Input: dimensioned drawing with shaded views. Units: mm. Origin: part minimum x, y, z. A direction names the side the tool comes from. Round coordinates to 2 decimals unless told otherwise and drop trailing zeros. Order: outer loops, then holes, each group sorted by start corner. A loop starts at its lowest first (then second) coordinate and runs counter-clockwise, first axis right, second up. Notation, with made-up numbers: M -31,51.25 L 13,51.25 A13 cw 13,55.25 Z; hole C -28,-1.75 d3. An arc over 180 degrees is marked long. Use CSV: the item, a comma, the result in double quotes. Start each with the question number.
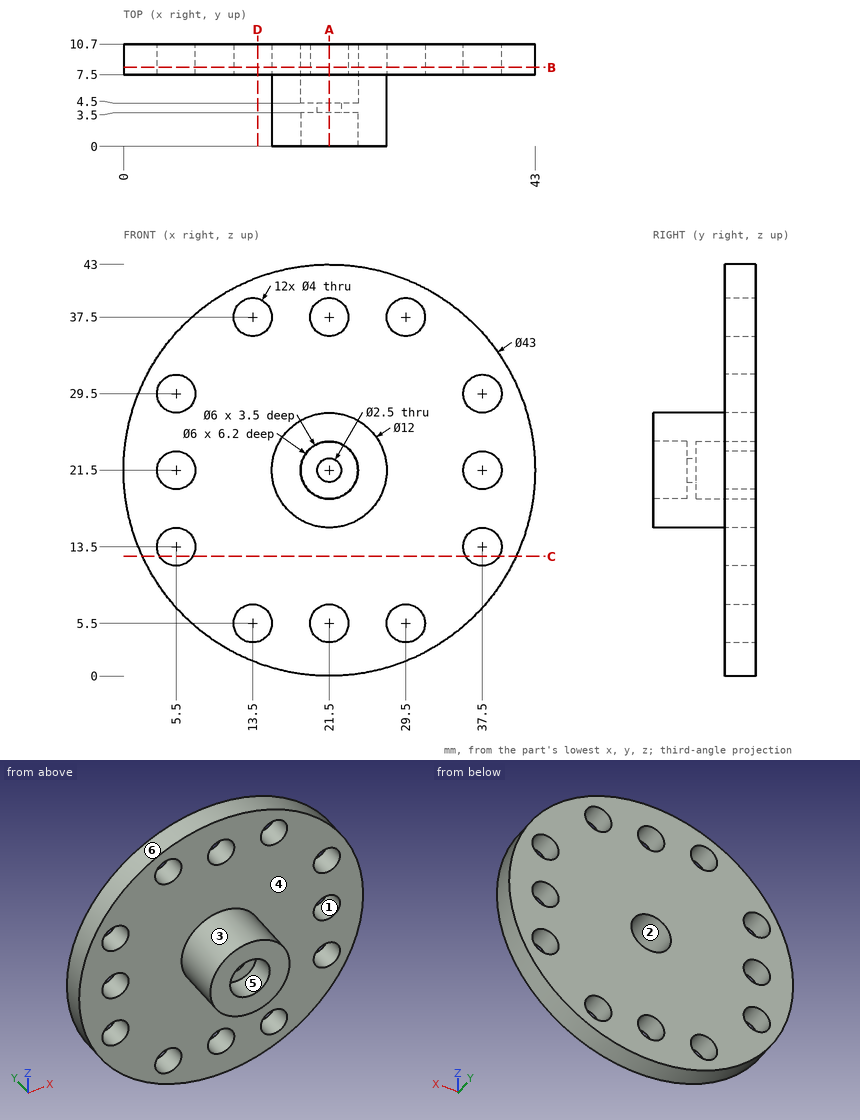
(1) Contact query for flat-ended pins moving along their axis: P1, Ø6, axis at x = 21, y = 1, coming from the +Z side; P2, Ø4.5, axis at x = 29.5, z = 5.5, coming from the -Y side; P3, Ø2.5, axis at x = 37.5, z = 13.5, coming from the -Y side; P4, Ø3, axis at y = 9.5, z = 31, coming from the -X side. Output: stop coordinate, or through.
(2) Reachability of the marked faces 1, 2 and 3 from +Z, -Z, +X, -X, +Y, -Y: full face, straight path, thin tool, end or side. Return the list, or none.
(3) Section D-D on x = 14. Return loops of the section in (y, z).
(4) Section B-B on y = 8.25. Give the number of separate pieces and of enclosed holes in the cut face, plus the area to 3 significant figures.
(5) Draft query along X for the marked faces 4, 5 and 6. Return one class per face: pulls with the +X half, pulls with the -X half, needs draft (parallel to the pull), parting line crosses it, or undercut.
(6) Section A-A on x = 21.5. Return loops of the section in (y, z).
(7) Section C-C on z = 12.5. Return loops of the section in (x, y).
(8) Line query: line 1 along X through (y, z) = (9, 21.5); line 2 along X through (y, z) = (9.5, 29.5). Output: solid intervals per line, ascending.
Results below:
1,P1,"stops at z = 27.5"
1,P2,"stops at y = 7.5"
1,P3,"passes through"
1,P4,"stops at x = 1.54"
2,face 1,"+Y, -Y"
2,face 2,"+Y"
2,face 3,"-Y"
3,outline,"M 7.5,1.35 L 10.7,1.35 L 10.7,3.56 L 7.5,3.56 Z; M 7.5,7.44 L 10.7,7.44 L 10.7,35.56 L 7.5,35.56 Z; M 7.5,39.44 L 10.7,39.44 L 10.7,41.65 L 7.5,41.65 Z"
4,separate pieces,"1"
4,enclosed holes,"13"
4,area,"1,270 mm2"
5,face 4,"needs draft"
5,face 5,"undercut"
5,face 6,"parting line crosses it"
6,outline,"M 0,15.5 L 7.5,15.5 L 7.5,7.5 L 10.7,7.5 L 10.7,18.5 L 4.5,18.5 L 4.5,20.25 L 3.5,20.25 L 3.5,18.5 L 0,18.5 Z; M 0,24.5 L 3.5,24.5 L 3.5,22.75 L 4.5,22.75 L 4.5,24.5 L 10.7,24.5 L 10.7,35.5 L 7.5,35.5 L 7.5,27.5 L 0,27.5 Z; M 7.5,0 L 10.7,0 L 10.7,3.5 L 7.5,3.5 Z; M 7.5,39.5 L 10.7,39.5 L 10.7,43 L 7.5,43 Z"
7,outline,"M 1.97,7.5 L 3.77,7.5 L 3.77,10.7 L 1.97,10.7 Z; M 7.23,7.5 L 35.77,7.5 L 35.77,10.7 L 7.23,10.7 Z; M 39.23,7.5 L 41.03,7.5 L 41.03,10.7 L 39.23,10.7 Z"
8,line 1,"x = 0 to 3.5, 7.5 to 18.5, 24.5 to 35.5, 39.5 to 43"
8,line 2,"x = 1.54 to 3.5, 7.5 to 35.5, 39.5 to 41.46"
